Autodesk Inventor part; units mm, degrees
ref_plane "YZ Plane" through (0, 0, 0) normal (1, 0, 0) x (0, 1, 0)
ref_plane "XZ Plane" through (0, 0, 0) normal (0, 1, 0) x (-1, 0, 0)
ref_plane "XY Plane" through (0, 0, 0) normal (0, 0, 1) x (1, 0, 0)
sketch "Sketch1" plane through (0, 0, 0) normal (0, 1, 0) x (-1, 0, 0)
  line L0 (0, 12.4728) -> (0, -12.4728) construction
  line L1 (2.135, 0) -> (-2.135, 0) construction
  line L2 (16, 20) -> (-16, 20)
  line L3 (-20, 16) -> (-20, -16)
  line L4 (-16, -20) -> (16, -20)
  line L5 (20, -16) -> (20, 16)
  arc A0 (-16, 20) -> (-20, 16) centre (-16, 16) ccw
  arc A1 (-20, -16) -> (-16, -20) centre (-16, -16) ccw
  arc A2 (16, -20) -> (20, -16) centre (16, -16) ccw
  arc A3 (20, 16) -> (16, 20) centre (16, 16) ccw
  point P0 (0, 0)
  point P1 (0, 0)
  dimension "d1" = 4
  dimension "d2" = 4
  dimension "d3" = 40
extrude "Extrusion1" add sketch "Sketch1" along normal blind 300
sketch "Sketch2" plane through (20, 0, 16) normal (1, 0, 0) x (0, 0, -1)
  line L0 (36, 0) -> (-4, 40)
  line L1 (-4, 40) -> (-4, 0)
  line L2 (-4, 0) -> (36, 0)
  line L3 (-4, 300) -> (-4, 260)
  line L4 (-4, 260) -> (36, 300)
  line L5 (36, 300) -> (-4, 300)
  line L6 (-4, 0) -> (-4, 300)
  line L7 (36, 0) -> (36, 300)
  point P0 (16, 0)
  dimension "d6" = 45
  dimension "d7" = 45
extrude "Extrusion2" cut sketch "Sketch2" against normal through all contours L2 L1 L0 | L4 L3 L5
properties part number "item40x40_1000"
CAD build for the part. Positions are in the model's coordinates, mm. Coordinates: 2 decimals unless noted, no trailing zeros. Order: outer loops, then holes, each group sorted by start corner. A loop starts at its lowest first (then second) coordinate and runs counter-clockwise, first axis right, second up. Notation, with made-up numbers: (72.5, 83.25) -> (114.5, 83.25) arc R32 cw to (114.5, 115.25) -> close; hole circle Ø8 at (21, 67). An arc over 180 degrees is marked (long way). Use one line per item in the form item = value. Start each with the question number.
1) Drill centre lines: L1, parallel to Y at x = -5, z = 16; L2, parallel to Y at x = 14, z = -16; L3, parallel to X at y = 246, z = -17. Where is each one in solid material? Low to high. Write a range as [from, to].
2) Band-saw the part on C-C on x = 6. Give the cut face in (y, z), then the cut area to 3 significant figures.
3) Band-saw the part on A-A on z = 0.5. Give the cut face in (x, y), then the cut area to 3 significant figures.
4) Band-saw the part on B-B on y = 32. Give the cut face in (x, z), then the cut area to 3 significant figures.
5) Drop flat-ended pins along their axis: pin 1 (10 mm diameter, centred on x = -2, z = -1.5, fed in from -Y); pin 2 (10 mm diameter, centred on x = -0.5, z = 8, fed in from -Y); pin 3 (8 mm diameter, centred on x = 5.5, z = 6.5, fed in from -Y). Give the stop position or say it passes through.
Entries:
q1.L1 = [36, 264]
q1.L2 = [4, 296]
q1.L3 = [-19.87, 19.87]
q2.outline = (0, -20) -> (300, -20) -> (260, 20) -> (40, 20) -> close
q2.area = 10,400 mm2
q3.outline = (-20, 20.5) -> (20, 20.5) -> (20, 279.5) -> (-20, 279.5) -> close
q3.area = 10,400 mm2
q4.outline = (-20, -16) arc R4 ccw to (-16, -20) -> (16, -20) arc R4 ccw to (20, -16) -> (20, 12) -> (-20, 12) -> close
q4.area = 1,270 mm2
q5.pin_1 = 13.5
q5.pin_2 = 23
q5.pin_3 = 22.5
